Verification items for the finished model (mm, model axes). A direction names the side the tool comes from. Round coordinates to 2 decimals unless told otherwise and drop trailing zeros. Order: outer loops, then holes, each group sorted by start corner. A loop starts at its lowest first (then second) coordinate and runs counter-clockwise, first axis right, second up. Notation, with made-up numbers: (30.5, -39.5) -> (48.5, -39.5) arc R30 ccw to (48.5, -15.5) -> close; hole circle Ø3 at (89, 85). An arc over 180 degrees is marked (long way). Put each result on its own line as item: value.
from build123d import *

# Parameters (mm, degrees)
SKETCH1_W           = 25
SKETCH1_H           = 135.5
BOSS_EXTRUDE1_DEPTH = 1.5
SKETCH2_R           = 5
CUT_EXTRUDE1_DEPTH  = 137.108412672
CHAMFER1_SIZE       = 5
SKETCH3_W           = 9.5
SKETCH3_H           = 4
CUT_EXTRUDE2_DEPTH  = 137.108412672


with BuildPart() as part:
    # Sketch1 → Boss-Extrude1 (new, symmetric)
    with BuildSketch(Plane.XY):
        with Locations((0, 67.75)):
            Rectangle(SKETCH1_W, SKETCH1_H)
    extrude(amount=BOSS_EXTRUDE1_DEPTH, both=True)

    # Sketch2 → Cut-Extrude1 (cut, through all)
    with BuildSketch(Plane.XY.offset(1.5)):
        with Locations((0, 118)):
            Circle(SKETCH2_R)
    extrude(amount=-CUT_EXTRUDE1_DEPTH, mode=Mode.SUBTRACT)

    # Chamfer1
    chamfer1_edges = [part.edges().sort_by_distance(p)[0] for p in [
        (-12.5, 135.5, 0),
        (12.5, 135.5, 0),
    ]]
    chamfer(chamfer1_edges, length=CHAMFER1_SIZE)

    # Sketch3 → Cut-Extrude2 (cut, through all)
    with BuildSketch(Plane.XY.offset(1.5)):
        with Locations((-7.75, 2)):
            Rectangle(SKETCH3_W, SKETCH3_H)
        with Locations((7.75, 2)):
            Rectangle(SKETCH3_W, SKETCH3_H)
    extrude(amount=-CUT_EXTRUDE2_DEPTH, mode=Mode.SUBTRACT)


solid = part.part
Item 1: Release check for a two-part mould opening along Y. For faces 1 (the flat face through (0, 135.5, 0)), 2 (the flat face through (3, 2, 0)), 3 (the cylindrical face through (-1.08, 113.12, 0.02)), 4 (the flat face through (-8, 4, 0)) record: +Y half, -Y half, draft (parallel to the pull), parting line (faces both ways), or undercut.
Check sheet entries:
face 1: +Y half
face 2: draft
face 3: undercut
face 4: -Y half
Item 2: Section check C-C on z = -1. Record the boundary of the cut face in (x, y).
Check sheet entries:
outline: (-12.5, 4) -> (-3, 4) -> (-3, 0) -> (3, 0) -> (3, 4) -> (12.5, 4) -> (12.5, 130.5) -> (7.5, 135.5) -> (-7.5, 135.5) -> (-12.5, 130.5) -> close; hole circle Ø10 at (0, 118)
Item 3: Section check A-A on y = 118. Record the boundary of the cut face in (x, z).
Check sheet entries:
outline: (-12.5, -1.5) -> (-5, -1.5) -> (-5, 1.5) -> (-12.5, 1.5) -> close; (5, -1.5) -> (12.5, -1.5) -> (12.5, 1.5) -> (5, 1.5) -> close
Item 4: Material ranges on L1, parallel to Y at x = 0, z = -0.7; L2, parallel to Y at x = 5.25, z = 1.45; L3, parallel to Y at x = 3.5, z = -0.7, recorded low to high. Write a range as [from, to].
Check sheet entries:
L1: y = [0, 113], [123, 135.5]
L2: y = [4, 135.5]
L3: y = [4, 114.43], [121.57, 135.5]
Item 5: Section check B-B on x = 0. Record the boundary of the cut face in (y, z), then the cut area to 4 significant figures.
Check sheet entries:
outline: (0, -1.5) -> (113, -1.5) -> (113, 1.5) -> (0, 1.5) -> close; (123, -1.5) -> (135.5, -1.5) -> (135.5, 1.5) -> (123, 1.5) -> close
area: 376.5 mm^2
Item 6: Gauge pin test, flat ends, axial feed: pin 1 Ø8 at (x, y) = (0, 118) entering from +Z; pin 2 Ø1.5 at (y, z) = (3, 0) entering from -X. Record the tip position at first contact, or that the pin passes through.
Check sheet entries:
pin 1: passes through
pin 2: stops at x = -3
Item 7: Tool access check on faces 5 (the flat face through (-3, 2, 0)), 6 (the flat face through (0, 0, 0)), 7 (the flat face through (8, 4, 0)). Record the directions out of +Z, -Z, +X, -X, +Y, -Y that give a thin tool (end or side, any length) a straight path to the whole face; none if there is none.
Check sheet entries:
face 5: +Z, -Z, -X, -Y
face 6: +Z, -Z, +X, -X, -Y
face 7: +Z, -Z, +X, -Y
